Geometry: see drawing. Coordinates: mm, zero at the bounding-box minimum. A direction names the side the tool comes from. Coordinates: 2 decimals unless noted, no trailing zeros. Loops run counter-clockwise (first coordinate to the right, second up) from the corner with the lowest first, then second, coordinate; pieces in that order, holes last. Notation, with made-up numbers: (37, -29) -> (78, -29) arc R23 ccw to (78, 7) -> close; hole circle Ø3 at (89, -5). An arc over 180 degrees is marked (long way). One line per item, written item: value. Start each with the question number.
Item 1: Mould query, pull axis X, two halves, no side actions, for the marked faces 3, 4 and 5. Classes: +X half, -X half, draft (parallel to the pull), parting line (faces both ways), or undercut.
Item 2: Contact query for a flat-ended pin moving along its axis: pin 1 Ø0.5 at (y, z) = (1.5, 0.5) entering from +X. Output: stop coordinate, or through.
Item 3: Set-up query: the marked faces 1 and 2. Return all of +Z, -Z, +X, -X, +Y, -Y with unobstructed straight access to the full face (end or side cutting, diameter ignored); none if empty.
Item 4: Ray query, probe 1 along Y at (x, z) = (5, 0.85); probe 2 along X at (y, z) = (6.75, 0.7) (1 decimal); probe 3 along X at (y, z) = (5.5, 0.2) (1 decimal). Return the intervals inside material, ascending. Write a range as from..to.
Item 5: Section query D-D on x = 6.25. Return loops of the section in (y, z).
Item 6: Section query C-C on x = 4.5. Return loops of the section in (y, z).
Item 7: Section query B-B on x = 8. Return loops of the section in (y, z).
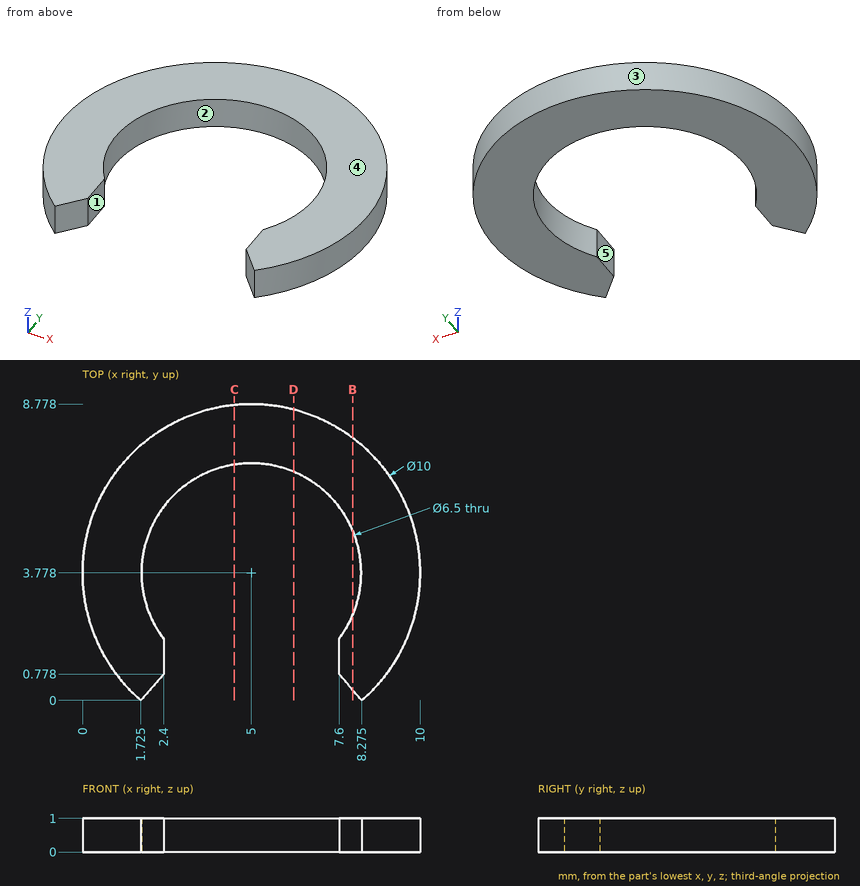
Reply:
1. face 3: parting line
1. face 4: draft
1. face 5: undercut
2. pin 1: stops at x = 9.57
3. face 1: +Z, -Z, -Y
3. face 2: +Z, -Z
4. probe 1: y = 7.03..8.78
4. probe 2: x = 1..3.7, 6.3..9
4. probe 3: x = 0.3..2.2, 7.8..9.7
5. outline: (6.78, 0) -> (8.62, 0) -> (8.62, 1) -> (6.78, 1) -> close
6. outline: (6.99, 0) -> (8.75, 0) -> (8.75, 1) -> (6.99, 1) -> close
7. outline: (0.32, 0) -> (2.53, 0) -> (2.53, 1) -> (0.32, 1) -> close; (5.03, 0) -> (7.78, 0) -> (7.78, 1) -> (5.03, 1) -> close
